from build123d import *

# Parameters (mm, degrees)
SKETCH1_W                  = 254
SKETCH1_H                  = 127
SKETCH1_W_2                = 38.608
SKETCH1_H_2                = 3.556
SKETCH1_W_3                = 3.556
SKETCH1_H_3                = 38.608
BOSS_EXTRUDE1_DEPTH        = 2.54
F_7_0_201_DIAMETER_HOLE1_D = 5.1054
SHELL1_T                   = -0.1016


with BuildPart() as part:
    # Sketch1 → Boss-Extrude1 (new body)
    with BuildSketch(Plane(origin=(0, 0, 0), x_dir=(1, 0, 0), z_dir=(0, 1, 0))):
        with Locations((127, 0)):
            Rectangle(SKETCH1_W, SKETCH1_H)
        with Locations((27.686, 56.896)):
            Rectangle(SKETCH1_W_2, SKETCH1_H_2, mode=Mode.SUBTRACT)
        with Locations((204.216, 56.896)):
            Rectangle(SKETCH1_W_2, SKETCH1_H_2, mode=Mode.SUBTRACT)
        with Locations((6.604, 34.036)):
            Rectangle(SKETCH1_W_3, SKETCH1_H_3, mode=Mode.SUBTRACT)
    boss_extrude1 = extrude(amount=BOSS_EXTRUDE1_DEPTH)

    # #7 (0.201) Diameter Hole1 (through all)
    with Locations(Plane(origin=(30.48, 2.54, 7.9756), x_dir=(0, 0, 1), z_dir=(0, 1, 0))):
        with Locations((0, 0), (0, 41.91)):
            f_7_0_201_diameter_hole1 = Hole(F_7_0_201_DIAMETER_HOLE1_D / 2)

    # Mirror1: Boss-Extrude1, #7 (0.201) Diameter Hole1 across plane
    add(boss_extrude1.mirror(Plane(origin=(0, 2.54, 63.5), x_dir=(1, 0, 0), z_dir=(0, 0, -1))))
    add(f_7_0_201_diameter_hole1.mirror(Plane(origin=(0, 2.54, 63.5), x_dir=(1, 0, 0), z_dir=(0, 0, -1))), mode=Mode.SUBTRACT)

    # Shell1
    shell1_openings = [part.faces().sort_by_distance(p)[0] for p in [
        (30.48, 2.54, 121.5771),
    ]]
    offset(amount=SHELL1_T, openings=shell1_openings, kind=Kind.INTERSECTION)


solid = part.part
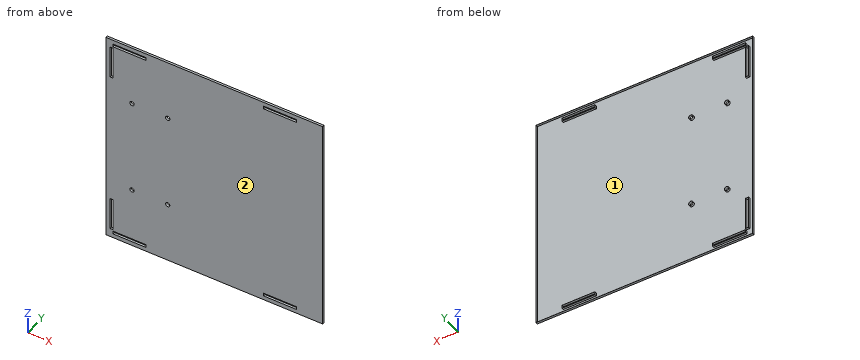
Design review of the part built by this model. Coordinates are the model's own, in mm. Face numbers are marked on the shaded views. Coordinates: 2 decimals unless noted, no trailing zeros. Loops run counter-clockwise (first coordinate to the right, second up) from the corner with the lowest first, then second, coordinate; pieces in that order, holes last.
Item 1: Add section B-B (x = 16). Write out the cut boundary in (y, z), and give its area (3 significant figures).
Completed:
outline: (0, -63.5) - (2.54, -63.5) - (2.54, -63.4) - (0.1, -63.4) - (0.1, -58.78) - (2.54, -58.78) - (2.54, -58.67) - (0, -58.67) - close; (0, -55.12) - (2.54, -55.12) - (2.54, -55.02) - (0.1, -55.02) - (0.1, 182.02) - (2.54, 182.02) - (2.54, 182.12) - (0, 182.12) - close; (0, 185.67) - (2.54, 185.67) - (2.54, 185.78) - (0.1, 185.78) - (0.1, 190.4) - (2.54, 190.4) - (2.54, 190.5) - (0, 190.5) - close
area: 26.6 mm2
Item 2: Add section A-A (z = -25). Write out the cut boundary in (x, y).
Completed:
outline: (0, 0) - (4.83, 0) - (4.83, 2.54) - (4.72, 2.54) - (4.72, 0.1) - (0.1, 0.1) - (0.1, 2.54) - (0, 2.54) - close; (8.38, 0) - (254, 0) - (254, 2.54) - (253.9, 2.54) - (253.9, 0.1) - (8.48, 0.1) - (8.48, 2.54) - (8.38, 2.54) - close
Item 3: Draft analysis for pull direction Z (two halves, no side actions). For the marked faces 1 and 2, state which applies: pulls with the +Z half, pulls with the -Z half, needs draft (parallel to the pull), parting line crosses it, or undercut.
Completed:
face 1: undercut
face 2: needs draft
Item 4: Add section D-D (z = 22). Write out the cut boundary in (x, y), and give its area (3 significant figures).
Completed:
outline: (0, 0) - (254, 0) - (254, 2.54) - (253.9, 2.54) - (253.9, 0.1) - (0.1, 0.1) - (0.1, 2.54) - (0, 2.54) - close
area: 26.3 mm2
Item 5: Add section C-C (x = 139). Write out the cut boundary in (y, z), and give its area (3 significant figures).
Completed:
outline: (0, -63.5) - (2.54, -63.5) - (2.54, -63.4) - (0.1, -63.4) - (0.1, 190.4) - (2.54, 190.4) - (2.54, 190.5) - (0, 190.5) - close
area: 26.3 mm2
